Source: CAD feature listing. Evaluate the final solid. Frame: model axes, mm. Round coordinates to 2 decimals unless told otherwise and drop trailing zeros. Loops run counter-clockwise (first coordinate to the right, second up) from the corner with the lowest first, then second, coordinate; pieces in that order, holes last. Notation, with made-up numbers: M 79,58.5 L 101,58.5 A20 ccw 101,81.5 Z; hole C 77.25,-12.5 d3. An arc over 180 degrees is marked long. Answer as a JSON object with one key per item and string values.
from build123d import *

# Parameters (mm, degrees)
F0_R     = 2.5
F0_R_2   = 3.5
F1_DEPTH = 3


with BuildPart() as f1:
    # F0 (on Top) → F1 (new body)
    with BuildSketch(Plane.XY):
        with BuildLine():
            Line((0, 18.81966), (0, 5))
            ThreePointArc((0, 5), (1.464466, 1.464466), (5, 0))
            Line((5, 0), (62.5, 0))
            ThreePointArc((62.5, 0), (66.035534, 1.464466), (67.5, 5))
            Line((67.5, 5), (67.5, 17.810844))
            ThreePointArc((67.5, 17.810844), (67.080229, 19.816211), (65.891401, 21.484861))
            Line((65.891401, 21.484861), (36.436481, 48.674017))
            ThreePointArc((36.436481, 48.674017), (34.865783, 49.65672), (33.045081, 50))
            Line((33.045081, 50), (18.09017, 50))
            ThreePointArc((18.09017, 50), (15.461514, 49.253254), (13.618034, 47.236068))
            Line((13.618034, 47.236068), (0.527864, 21.055728))
            ThreePointArc((0.527864, 21.055728), (0.133755, 19.968425), (0, 18.81966))
        make_face()
        with Locations((5, 10)):
            Circle(F0_R, mode=Mode.SUBTRACT)
        with Locations((25, 10)):
            Circle(F0_R, mode=Mode.SUBTRACT)
        with Locations((62.5, 10)):
            Circle(F0_R_2, mode=Mode.SUBTRACT)
        with Locations((25, 30)):
            Circle(F0_R, mode=Mode.SUBTRACT)
        with Locations((25, 45)):
            Circle(F0_R, mode=Mode.SUBTRACT)
    extrude(amount=F1_DEPTH)


solid = f1.part
Item 1: Section A-A on y = 10. Return the cut outline in (x, z).
Answer sheet:
{"outline": "M 0,0 L 2.5,0 L 2.5,3 L 0,3 Z; M 7.5,0 L 22.5,0 L 22.5,3 L 7.5,3 Z; M 27.5,0 L 59,0 L 59,3 L 27.5,3 Z; M 66,0 L 67.5,0 L 67.5,3 L 66,3 Z"}
Item 2: Line query: probe 1 along Y at (x, z) = (25, 2.35); probe 2 along Y at (x, z) = (26, 1.85); probe 3 along X at (y, z) = (9, 2.3). Output: solid intervals per line, ascending. Write a range as from..to.
Answer sheet:
{"probe 1": "y = 0..7.5, 12.5..27.5, 32.5..42.5, 47.5..50", "probe 2": "y = 0..7.71, 12.29..27.71, 32.29..42.71, 47.29..50", "probe 3": "x = 0..2.71, 7.29..22.71, 27.29..59.15, 65.85..67.5"}
Item 3: Pull-direction query (X, two-part tool) for faces 1 (the flat face through (0, 12, 1)), 2 (the cylindrical face through (6.15, 7.78, 1.48)), 3 (the flat face through (26, 50, 1)); classes: pulls with the +X half, pulls with the -X half, needs draft (parallel to the pull), parting line crosses it, or undercut.
Answer sheet:
{"face 1": "pulls with the -X half", "face 2": "undercut", "face 3": "needs draft"}
Item 4: Contact query for a flat-ended pin moving along its axis: pin 1 Ø3 at (x, y) = (25, 10) entering from +Z. Output: stop coordinate, or through.
Answer sheet:
{"pin 1": "passes through"}
Item 5: Section B-B on z = 0.75. Return the cut outline in (x, y).
Answer sheet:
{"outline": "M 0,5 A5 ccw 5,0 L 62.5,0 A5 ccw 67.5,5 L 67.5,17.81 A5 ccw 65.89,21.48 L 36.44,48.67 A5 ccw 33.05,50 L 18.09,50 A5 ccw 13.62,47.24 L 0.53,21.06 A5 ccw 0,18.82 Z; hole C 5,10 d5; hole C 25,10 d5; hole C 25,30 d5; hole C 25,45 d5; hole C 62.5,10 d7"}
Item 6: Section D-D on y = 23. Return the cut outline in (x, z), then the cut area to 3 significant figures.
Answer sheet:
{"outline": "M 1.5,0 L 64.25,0 L 64.25,3 L 1.5,3 Z", "area": "188 mm²"}
Item 7: Section C-C on y = 30. Return the cut outline in (x, z), then the cut area to 3 significant figures.
Answer sheet:
{"outline": "M 5,0 L 22.5,0 L 22.5,3 L 5,3 Z; M 27.5,0 L 56.67,0 L 56.67,3 L 27.5,3 Z", "area": "140 mm²"}
